Here's how the part is built. I have some questions about the finished solid (model axes, mm). A direction names the side the tool comes from. Round coordinates to 2 decimals unless told otherwise and drop trailing zeros. Loops run counter-clockwise (first coordinate to the right, second up) from the corner with the lowest first, then second, coordinate; pieces in that order, holes last. Notation, with made-up numbers: (-35, 55) - (10, 55) arc R24 ccw to (10, 82) - close; hole circle Ø4 at (10.5, 20.5). An arc over 180 degrees is marked (long way). Return JSON: item names as keys, results as strings. Group by question number.
```python
from build123d import *

# Parameters (mm, degrees)
SKETCH_1_W               = 45
SKETCH_1_H               = 20
EXTRUDE_1_DEPTH          = 3
SKETCH_2_R               = 7.5
EXTRUDE_2_DEPTH          = 13
SKETCH_3_R               = 1.75
CUT_EXTRUDE_1_DEPTH      = 14
CUT_EXTRUDE_1_DEPTH_BACK = 4
SKETCH_4_R               = 6.5
CUT_EXTRUDE_2_DEPTH      = 2


with BuildPart() as part:
    # 草图1 → 凸台-拉伸1 (new body)
    with BuildSketch(Plane.XY):
        Rectangle(SKETCH_1_W, SKETCH_1_H)
    extrude(amount=EXTRUDE_1_DEPTH)

    # 草图2 → 凸台-拉伸2 (add)
    with BuildSketch(Plane.XY.offset(3)):
        with Locations((12.5, 0)):
            Circle(SKETCH_2_R)
        with Locations((-12.5, 0)):
            Circle(SKETCH_2_R)
    extrude(amount=EXTRUDE_2_DEPTH)

    # 草图3 → 切除-拉伸1 (cut, two sides)
    with BuildSketch(Plane.XY.offset(3)) as cut_extrude_1_sk:
        with Locations((20.2, 7)):
            Circle(SKETCH_3_R)
        with Locations((-20.2, -7)):
            Circle(SKETCH_3_R)
    extrude(amount=CUT_EXTRUDE_1_DEPTH, mode=Mode.SUBTRACT)
    extrude(cut_extrude_1_sk.sketch, amount=-CUT_EXTRUDE_1_DEPTH_BACK, mode=Mode.SUBTRACT)

    # 草图4 → 切除-拉伸2 (cut)
    with BuildSketch(Plane.XY.offset(16)):
        with Locations((-12.5, 0)):
            Circle(SKETCH_4_R)
        with Locations((12.5, 0)):
            Circle(SKETCH_4_R)
    extrude(amount=-CUT_EXTRUDE_2_DEPTH, mode=Mode.SUBTRACT)


solid = part.part
```
Q1. If we mould it in two halves opening along Y, with no side actions, what happens to faces 1 (the flat face through (0, -10, 1)), 2 (the flat face through (-13, 7, 16)), 3 (the cylindrical face through (18.7, 1.95, 15.01)), 4 (the cylindrical face through (5, 0, 9))? For each: +Y half, -Y half, draft (parallel to the pull), parting line (faces both ways), or undercut.
Q2. Imagine slicing it at A-A, the plane y = 0. List the corners of the cut face in (x, z) for me.
Q3. Imagine slicing it at D-D, the plane z = 1.75. List the corners of the cut face in (x, y) for me, and give its area (3 significant figures).
Q4. Will these pins go through, and if not, where does the flat tip stop? pin 1 Ø6 at (x, y) = (0.5, 0.5) entering from +Z; pin 2 Ø1 at (y, z) = (0.5, 11.5) entering from -X; pin 3 Ø4 at (x, y) = (-14.5, 1.5) entering from +Z.
Q5. Imagine slicing it at B-B, the plane z = 14.75. List the corners of the cut face in (x, y) for me, and give its area (3 significant figures).
Q6. Please list where these lines run through material, in increasing order: line 1 (Y direction, x = -12.5, z = 15.4); line 2 (X direction, y = 4, z = 14.75); line 3 (Z direction, x = 3.5, y = 4.5).
Q7. Imagine slicing it at C-C, the plane x = 12.5. List the corners of the cut face in (y, z) for me.
Q8. For faces 5 (the flat face through (-22.5, 0, 1)), 6 (the flat face through (-13, 0, 14)), which set-ups out of +Z, -Z, +X, -X, +Y, -Y let a thin tool reach every point of the face, with its end or its side?
Output values:
{
 "1": {"face 1": "-Y half", "face 2": "draft", "face 3": "undercut", "face 4": "parting line"},
 "2": {"outline": "(-22.5, 0) - (22.5, 0) - (22.5, 3) - (20, 3) - (20, 16) - (19, 16) - (19, 14) - (6, 14) - (6, 16) - (5, 16) - (5, 3) - (-5, 3) - (-5, 16) - (-6, 16) - (-6, 14) - (-19, 14) - (-19, 16) - (-20, 16) - (-20, 3) - (-22.5, 3) - close"},
 "3": {"outline": "(-22.5, -10) - (22.5, -10) - (22.5, 10) - (-22.5, 10) - close; hole circle Ø3.5 at (-20.2, -7); hole circle Ø3.5 at (20.2, 7)", "area": "881 mm^2"},
 "4": {"pin 1": "stops at z = 3", "pin 2": "stops at x = -20", "pin 3": "stops at z = 14"},
 "5": {"outline": "circle Ø15 at (-12.5, 0); circle Ø15 at (12.5, 0); hole circle Ø13 at (-12.5, 0); hole circle Ø13 at (12.5, 0)", "area": "88.0 mm^2"},
 "6": {"line 1": "y = -7.5 to -6.5, 6.5 to 7.5", "line 2": "x = -18.84 to -17.62, -7.38 to -6.16, 6.16 to 7.38, 17.62 to 18.84", "line 3": "z = 0 to 3"},
 "7": {"outline": "(-10, 0) - (10, 0) - (10, 3) - (7.5, 3) - (7.5, 16) - (6.5, 16) - (6.5, 14) - (-6.5, 14) - (-6.5, 16) - (-7.5, 16) - (-7.5, 3) - (-10, 3) - close"},
 "8": {"face 5": "+Z, -Z, -X, +Y, -Y", "face 6": "+Z"}
}
